```python
from build123d import *

# Parameters (mm, degrees)
SKETCH1_W           = 104
SKETCH1_H           = 140
BOSS_EXTRUDE1_DEPTH = 1
SKETCH2_W           = 1
SKETCH2_H           = 20
BOSS_EXTRUDE2_DEPTH = 15
SKETCH6_R           = 2
CUT_EXTRUDE1_DEPTH  = 30
FILLET3_R           = 10
FILLET4_R           = 10
FILLET5_R           = 10
FILLET6_R           = 10
SKETCH9_W           = 10
SKETCH9_H           = 1
BOSS_EXTRUDE5_DEPTH = 11
SKETCH10_R          = 1
CUT_EXTRUDE2_DEPTH  = 150.268214969
SKETCH12_R          = 1
CUT_EXTRUDE3_DEPTH  = 150.268214969
CUT_EXTRUDE4_DEPTH  = 12


with BuildPart() as part:
    # Sketch1 → Boss-Extrude1 (new body)
    with BuildSketch(Plane(origin=(0, 0, 0), x_dir=(1, 0, 0), z_dir=(0, 1, 0))):
        Rectangle(SKETCH1_W, SKETCH1_H)
    extrude(amount=BOSS_EXTRUDE1_DEPTH)

    # Sketch2 → Boss-Extrude2 (add)
    with BuildSketch(Plane(origin=(0, 1, 0), x_dir=(1, 0, 0), z_dir=(0, 1, 0))):
        with Locations((-10.719821852, -10)):
            Rectangle(SKETCH2_W, SKETCH2_H)
        with Locations((10.719821852, -10)):
            Rectangle(SKETCH2_W, SKETCH2_H)
    extrude(amount=BOSS_EXTRUDE2_DEPTH)

    # Sketch6 → Cut-Extrude1 (cut)
    with BuildSketch(Plane(origin=(11.219821852, 0, 0), x_dir=(0, 0, -1), z_dir=(1, 0, 0))):
        with Locations((-10, 9.5)):
            Circle(SKETCH6_R)
    extrude(amount=-CUT_EXTRUDE1_DEPTH, mode=Mode.SUBTRACT)

    # Fillet3
    fillet3_edges = [part.edges().sort_by_distance(p)[0] for p in [
        (10.719821852, 16, 20),
    ]]
    fillet(fillet3_edges, radius=FILLET3_R)

    # Fillet4
    fillet4_edges = [part.edges().sort_by_distance(p)[0] for p in [
        (10.719821852, 16, 0),
    ]]
    fillet(fillet4_edges, radius=FILLET4_R - 0.0001)  # a hair under: the kernel refuses the full size

    # Fillet5
    fillet5_edges = [part.edges().sort_by_distance(p)[0] for p in [
        (-10.719821852, 16, 20),
    ]]
    fillet(fillet5_edges, radius=FILLET5_R)

    # Fillet6
    fillet6_edges = [part.edges().sort_by_distance(p)[0] for p in [
        (-10.719821852, 16, 0),
    ]]
    fillet(fillet6_edges, radius=FILLET6_R - 0.0001)  # a hair under: the kernel refuses the full size

    # Sketch9 → Boss-Extrude5 (add)
    with BuildSketch(Plane.XZ):
        with Locations((46, -68.5)):
            Rectangle(SKETCH9_W, SKETCH9_H)
        with Locations((-46, -68.5)):
            Rectangle(SKETCH9_W, SKETCH9_H)
        with Locations((-46, 68.5)):
            Rectangle(SKETCH9_W, SKETCH9_H)
        with Locations((46, 68.5)):
            Rectangle(SKETCH9_W, SKETCH9_H)
    extrude(amount=BOSS_EXTRUDE5_DEPTH)

    # Sketch10 → Cut-Extrude2 (cut, through all)
    with BuildSketch(Plane(origin=(0, 0, -69), x_dir=(-1, 0, 0), z_dir=(0, 0, -1))):
        with Locations((46, -8)):
            Circle(SKETCH10_R)
        with Locations((46, -4)):
            Circle(SKETCH10_R)
    extrude(amount=-CUT_EXTRUDE2_DEPTH, mode=Mode.SUBTRACT)

    # Sketch12 → Cut-Extrude3 (cut, through all)
    with BuildSketch(Plane.XY.offset(69)):
        with Locations((46, -4)):
            Circle(SKETCH12_R)
        with Locations((46, -8)):
            Circle(SKETCH12_R)
    extrude(amount=-CUT_EXTRUDE3_DEPTH, mode=Mode.SUBTRACT)

    # Sketch13 → Cut-Extrude4 (cut)
    with BuildSketch(Plane(origin=(0, 1, 0), x_dir=(1, 0, 0), z_dir=(0, 1, 0))):
        Polygon((0, 70), (-36, 70), (-36, 60), (36, 60), (36, 70), align=None)
    extrude(amount=-CUT_EXTRUDE4_DEPTH, mode=Mode.SUBTRACT)


solid = part.part
```
The model under review builds one solid part; all positions refer to its coordinate system, in mm. A direction names the side the tool comes from. Round coordinates to 2 decimals unless told otherwise and drop trailing zeros. Loops run counter-clockwise (first coordinate to the right, second up) from the corner with the lowest first, then second, coordinate; pieces in that order, holes last. Notation, with made-up numbers: (17.25, 12.25) -> (71.25, 12.25) arc R3 ccw to (71.25, 16.25) -> close; hole circle Ø1 at (-34.75, 19). An arc over 180 degrees is marked (long way). Answer in a Markdown table with one row per item.
1) Tool access review of faces 4 (the flat face through (10.22, 7, 10)), 5 (the flat face through (45.9, -5.4, 69)), 6 (the flat face through (45.9, -5.4, -69)), 7 (the flat face through (11.22, 7, 10)), 8 (the flat face through (45.9, -5.4, 68)): name each direction out of +Z, -Z, +X, -X, +Y, -Y from which nothing blocks a thin tool from reaching the whole face with its end or side.
Taken from the geometry:
| item | result |
|---|---|
| face 4 | +Z, -Z, +Y |
| face 5 | +Z, +X, -X, -Y |
| face 6 | -Z, +X, -X, -Y |
| face 7 | +Z, -Z, +X, +Y |
| face 8 | +X, -X, -Y |
2) Consider section C-C, the plane x = 26.5. Write out the cut boundary in (y, z).
Taken from the geometry:
| item | result |
|---|---|
| outline | (0, -60) -> (1, -60) -> (1, 70) -> (0, 70) -> close |
3) Wall thickness on line 1 along Y through (x, z) = (46, 68.8); line 2 along Y through (x, z) = (14.5, -32): over which ranges is each line inside the solid? List them lowest first.
Taken from the geometry:
| item | result |
|---|---|
| line 1 | y = -11 to -9, -7 to -5, -3 to 1 |
| line 2 | y = 0 to 1 |
4) Consider section A-A, the plane y = 9.5. Write out the cut boundary in (x, z), plus the area to 3 significant figures.
Taken from the geometry:
| item | result |
|---|---|
| outline | (-11.22, 0.63) -> (-10.22, 0.63) -> (-10.22, 8) -> (-11.22, 8) -> close; (-11.22, 12) -> (-10.22, 12) -> (-10.22, 19.37) -> (-11.22, 19.37) -> close; (10.22, 0.63) -> (11.22, 0.63) -> (11.22, 8) -> (10.22, 8) -> close; (10.22, 12) -> (11.22, 12) -> (11.22, 19.37) -> (10.22, 19.37) -> close |
| area | 29.5 mm² |
5) Consider section B-B, the plane z = 49.5. Write out the cut boundary in (x, y), plus the area to 3 significant figures.
Taken from the geometry:
| item | result |
|---|---|
| outline | (-52, 0) -> (52, 0) -> (52, 1) -> (-52, 1) -> close |
| area | 104 mm² |
6) Draft analysis for pull direction X (two halves, no side actions). For faces 1 (the flat face through (-11.22, 7, 10)), 2 (the flat face through (-46.1, -5.4, 69)), 3 (the flat face through (-10.22, 7, 10)), state which applies: pulls with the +X half, pulls with the -X half, needs draft (parallel to the pull), parting line crosses it, or undercut.
Taken from the geometry:
| item | result |
|---|---|
| face 1 | pulls with the -X half |
| face 2 | needs draft |
| face 3 | undercut |
7) For pin 1 Ø3 at (x, y) = (48, -6) entering from +Z; pin 2 Ø0.5 at (x, y) = (11, 4.5) entering from +Z; pin 3 Ø6 at (x, z) = (-13.5, 3) entering from +Y, all flat-tipped, find the tip position at first contact; note any pin that passes through.
Taken from the geometry:
| item | result |
|---|---|
| pin 1 | stops at z = 69 |
| pin 2 | stops at z = 20 |
| pin 3 | stops at y = 14.63 |
